Design review of the part built by this model. Coordinates are the model's own, in mm. A direction names the side the tool comes from. Round coordinates to 2 decimals unless told otherwise and drop trailing zeros. Loops run counter-clockwise (first coordinate to the right, second up) from the corner with the lowest first, then second, coordinate; pieces in that order, holes last. Notation, with made-up numbers: (57.5, 45.5) - (67.5, 45.5) arc R32 ccw to (67.5, 73.5) - close; hole circle Ø3 at (7.5, 32.5). An arc over 180 degrees is marked (long way). Answer as CSV lines item,"result". Start each with the question number.
(1) Consider section C-C (x = -84). Give the boundary of the cut face in (y, z), and give its area (3 significant figures).
(2) Consider section D-D (y = -14). Give the boundary of the cut face in (x, z).
(3) Mouldability with a two-part tool opening along X and no side actions: class faces 1 (the flat face through (-2, -45, -20)), 2 (the flat face through (-170, -45, 0)), 3 (the flat face through (110, 5, 0)) as released by +X, released by -X, zero draft, split by the parting line, or undercut.
(4) For P1, Ø3, axis at x = 61, y = -34.5, coming from the -Z side; P2, Ø12, axis at x = 123, y = 13, coming from the +Z side; P3, Ø22, axis at y = 10, z = -3, coming from the +X side, all flat-tipped, find the tip position at first contact; note any pin that passes through.
(5) Consider section B-B (z = 2). Give the boundary of the cut face in (x, y).
(6) For faces 4 (the flat face through (-2, -7, -10)), 5 (the flat face through (-2, -5, 0)), 6 (the flat face through (150, -14, 0)), 7 (the flat face through (-150, -13, 0)), list the 3-axis set-ups (+Z, -Z, +X, -X, +Y, -Y) from which the entire face can be reached by the end or side of a thin tool; tool diameter is ignored.
(7) Consider section A-A (y = 2). Give the boundary of the cut face in (x, z).
(8) Wall thickness on L1, parallel to Y at x = -18.5, z = -2.5; L2, parallel to X at y = 3, z = -3; L3, parallel to Y at x = -154, z = 9.5: over which ranges is each line inside the solid? List them lowest first.
from build123d import *

# Parameters (mm, degrees)
SKETCH1_W           = 220
SKETCH1_H           = 20
BOSS_EXTRUDE1_DEPTH = 10
SKETCH2_W           = 340
SKETCH2_H           = 40
BOSS_EXTRUDE2_DEPTH = 20
FILLET1_R           = 3


with BuildPart() as part:
    # Sketch1 → Boss-Extrude1 (new, symmetric)
    with BuildSketch(Plane.XY):
        with BuildLine():
            Line((-150, -35), (150, -35))
            Line((150, -35), (150, 5))
            ThreePointArc((150, 5), (141.213203436, 26.213203436), (120, 35))
            Line((120, 35), (-120, 35))
            ThreePointArc((-120, 35), (-141.213203436, 26.213203436), (-150, 5))
            Line((-150, 5), (-150, -35))
        make_face()
        with Locations((0, 5)):
            Rectangle(SKETCH1_W, SKETCH1_H, mode=Mode.SUBTRACT)
    extrude(amount=BOSS_EXTRUDE1_DEPTH, both=True)

    # Sketch2 → Boss-Extrude2 (add)
    with BuildSketch(Plane.XZ.offset(35)):
        Rectangle(SKETCH2_W, SKETCH2_H)
    extrude(amount=BOSS_EXTRUDE2_DEPTH)

    # Fillet1
    fillet1_edges = [part.edges().sort_by_distance(p)[0] for p in [
        (150, -35, 0),
        (-150, -35, 0),
        (150, -15, 10),
        (141.213203436, 26.213203436, 10),
        (0, 35, 10),
        (-141.213203436, 26.213203436, 10),
        (170, -35, 0),
        (170, -45, -20),
        (0, -35, 20),
        (170, -45, 20),
        (-170, -35, 0),
        (-170, -45, 20),
        (0, -35, -20),
        (-170, -45, -20),
        (170, -55, 0),
        (0, -55, 20),
        (-170, -55, 0),
        (0, -55, -20),
        (-150, -15, 10),
        (-141.213203436, 26.213203436, -10),
        (0, 35, -10),
        (141.213203436, 26.213203436, -10),
        (150, -15, -10),
        (0, -35, -10),
        (-150, -15, -10),
        (0, -35, 10),
    ]]
    fillet(fillet1_edges, radius=FILLET1_R)


solid = part.part
Determined:
1,outline,"(-55, -17) arc R3 ccw to (-52, -20) - (-38, -20) arc R3 ccw to (-35, -17) - (-35, -13) arc R3 cw to (-32, -10) - (-5, -10) - (-5, 10) - (-32, 10) arc R3 cw to (-35, 13) - (-35, 17) arc R3 ccw to (-38, 20) - (-52, 20) arc R3 ccw to (-55, 17) - close; (15, -10) - (32, -10) arc R3 ccw to (35, -7) - (35, 7) arc R3 ccw to (32, 10) - (15, 10) - close"
1,area,"1,790 mm^2"
2,outline,"(-150, -7) arc R3 ccw to (-147, -10) - (147, -10) arc R3 ccw to (150, -7) - (150, 7) arc R3 ccw to (147, 10) - (-147, 10) arc R3 ccw to (-150, 7) - close"
3,face 1,"zero draft"
3,face 2,"released by -X"
3,face 3,"undercut"
4,P1,"stops at z = -19.24"
4,P2,"stops at z = 10"
4,P3,"stops at x = 150"
5,outline,"(-170, -52) arc R3 ccw to (-167, -55) - (167, -55) arc R3 ccw to (170, -52) - (170, -38) arc R3 ccw to (167, -35) - (153, -35) arc R3 cw to (150, -32) - (150, 5) arc R30 ccw to (120, 35) - (-120, 35) arc R30 ccw to (-150, 5) - (-150, -32) arc R3 cw to (-153, -35) - (-167, -35) arc R3 ccw to (-170, -38) - close; hole (-110, -5) - (110, -5) - (110, 15) - (-110, 15) - close"
6,face 4,"-Z, +X, -X, +Y"
6,face 5,"+Z, -Z"
6,face 6,"+Z, -Z, +X, +Y"
6,face 7,"+Z, -Z, -X, +Y"
7,outline,"(-150, -7) arc R3 ccw to (-147, -10) - (-110, -10) - (-110, 10) - (-147, 10) arc R3 ccw to (-150, 7) - close; (110, -10) - (147, -10) arc R3 ccw to (150, -7) - (150, 7) arc R3 ccw to (147, 10) - (110, 10) - close"
8,L1,"y = -55 to -5, 15 to 35"
8,L2,"x = -150 to -110, 110 to 150"
8,L3,"y = -55 to -35"
